```python
from build123d import *

# Parameters (mm, degrees)
CUT_EXTRUDE_1_DEPTH = 1.04
CHAMFER_1_SIZE      = 0.3


with BuildPart() as part:
    # 草图1 → 旋转1 (revolve)
    with BuildSketch(Plane.XY, mode=Mode.PRIVATE) as revolve_1_sk:
        with BuildLine():
            Line((0, 0), (0, 1.5))
            Line((0, 1.5), (-5, 1.5))
            Line((-5, 1.5), (-6, 1.8))
            Line((-6, 1.8), (-6, 2.85))
            ThreePointArc((-6, 2.85), (-6.924953874, 2.424670081), (-7.65, 1.71))
            Line((-7.65, 1.71), (-7.65, 0))
            Line((-7.65, 0), (0, 0))
        make_face()
    revolve(revolve_1_sk.sketch.rotate(Axis((0, 0, 0), (-1, 0, 0)), 90), axis=Axis((0, 0, 0), (-1, 0, 0)))

    # 草图4 → 切除-拉伸1 (cut)
    with BuildSketch(Plane.ZY.offset(7.65)):
        Polygon((0, 1.154700538), (-1, 0.577350269), (-1, -0.577350269), (0, -1.154700538), (1, -0.577350269), (1, 0.577350269), align=None)
    extrude(amount=-CUT_EXTRUDE_1_DEPTH, mode=Mode.SUBTRACT)

    # 倒角1
    chamfer_1_edges = [part.edges().sort_by_distance(p)[0] for p in [
        (0, 0, 1.5),
    ]]
    chamfer(chamfer_1_edges, length=CHAMFER_1_SIZE)

    # 草图6 → 切除-放样1 section 0
    with BuildSketch(Plane.ZY.offset(6.61), mode=Mode.PRIVATE) as loft_1_s0:
        with BuildLine():
            Line((0, 1.154700538), (-1, 0.577350269))
            Line((-1, 0.577350269), (-1, -0.577350269))
            Line((-1, -0.577350269), (0, -1.154700538))
            Line((0, -1.154700538), (1, -0.577350269))
            Line((1, -0.577350269), (1, 0.577350269))
            Line((1, 0.577350269), (0, 1.154700538))
        make_face()
    loft([Vertex(-6.40375, 0, 0), loft_1_s0.sketch], mode=Mode.SUBTRACT)


solid = part.part
```
Design review of the part built by this model. Coordinates are the model's own, in mm. A direction names the side the tool comes from. Give positions to 0.01 mm unless a question says otherwise; leave off trailing zeros. Order: outer loops, then holes, each group sorted by start corner. A loop starts at its lowest first (then second) coordinate and runs counter-clockwise, first axis right, second up. Notation, with made-up numbers: (13, -34) - (34, -34) arc R32 ccw to (34, -8) - close; hole circle Ø4 at (8.5, 37). An arc over 180 degrees is marked (long way). Use a Markdown table: item, result. Add a question column.
(1) Add section A-A on x = -4.25. Give the boundary of the cut face in (y, z).
(2) Add section B-B on z = -2.35. Give the boundary of the cut face in (x, y), then the cut area to 3 significant figures.
(3) Machinability: for faces 4 (the face through (-6.53, 0.54, -0.3)), 5 (the face through (0, 0, 0)), 6 (the face through (-6, 0, 2)), which of the approach directions +Z, -Z, +X, -X, +Y, -Y give a long, thin tool a straight path to every point of the face, cutting with its end or side? Answer none if there is none.
(4) Clearance check with flat-ended pins moving along their axes: P1, Ø0.8, axis at x = -7.5, y = 0, coming from the -Z side; P2, Ø3, axis at x = -4, z = -1, coming from the -Y side; P3, Ø1.5, axis at x = -2.5, z = 1.5, coming from the +Y side. State where each tip first meets the part, or that it passes through.
(5) Wall thickness on probe 1 along X at (y, z) = (-0.6, -0.9); probe 2 along Z at (x, y) = (-1.5, -0.2); probe 3 along X at (y, z) = (1.15, 1.6): over which ranges is each line inside the solid? List them lowest first. Write a range as [from, to].
(6) Add section C-C on y = 2.2. Give the boundary of the cut face in (x, z).
(7) Mouldability with a two-part tool opening along Z and no side actions: class faces 1 (the face through (-7.65, 1, -1)), 2 (the face through (-6.53, -0.01, 0.62)), 3 (the face through (-2.68, -0.45, -1.43)) as +Z half, -Z half, draft (parallel to the pull), parting line (faces both ways), or undercut.
Report:
| question | item | result |
|---|---|---|
| 1 | outline | circle Ø3 at (0, 0) |
| 2 | outline | (-6, -1.61) - (-6, 1.61) arc R1.78 ccw to start |
| 2 | area | 2.38 mm² |
| 3 | face 4 | -X |
| 3 | face 5 | +Z, -Z, +X, +Y, -Y |
| 3 | face 6 | +X |
| 4 | P1 | stops at z = -2.29 |
| 4 | P2 | stops at y = -1.57 |
| 4 | P3 | stops at y = 1.3 |
| 5 | probe 1 | x = [-6.6, 0] |
| 5 | probe 2 | z = [-1.49, 1.49] |
| 5 | probe 3 | x = [-7.44, -6] |
| 6 | outline | (-6, -1.81) - (-6, 1.81) arc R1.96 ccw to start |
| 7 | face 1 | draft |
| 7 | face 2 | undercut |
| 7 | face 3 | parting line |
